Geometry: final body of the model. Coordinates: model frame, mm. A direction names the side the tool comes from. Give positions to 0.01 mm unless a question says otherwise; leave off trailing zeros. Write each loop counter-clockwise with the first axis right and the second up, starting at its lowest first coordinate (ties: lowest second). Pieces come first, ordered by that corner, then holes.
from build123d import *

# Parameters (mm, degrees)
SKETCH1_W           = 75
SKETCH1_H           = 10
BOSS_EXTRUDE1_DEPTH = 100
SKETCH2_R           = 5
CUT_EXTRUDE1_DEPTH  = 10
FILLET1_R           = 10
SKETCH3_R           = 4
CUT_EXTRUDE2_DEPTH  = 192


with BuildPart() as part:
    # Sketch1 → Boss-Extrude1 (new body)
    with BuildSketch(Plane.XY):
        with Locations((112.5, -5)):
            Rectangle(SKETCH1_W, SKETCH1_H)
        with Locations((37.5, -5)):
            Rectangle(SKETCH1_W, SKETCH1_H)
        Polygon((150, 0), (150, -10), (160, -10), (160, 90), (150, 90), align=None)
        Polygon((-10, -10), (0, -10), (0, 0), (0, 90), (-10, 90), align=None)
    extrude(amount=BOSS_EXTRUDE1_DEPTH)

    # Sketch2 → Cut-Extrude1 (cut)
    with BuildSketch(Plane(origin=(0, 0, 0), x_dir=(1, 0, 0), z_dir=(0, 1, 0))):
        with Locations(Location((75, -50, 0), (0, 0, 270))):
            Circle(SKETCH2_R)
    extrude(amount=-CUT_EXTRUDE1_DEPTH, mode=Mode.SUBTRACT)

    # Fillet1
    fillet1_edges = [part.edges().sort_by_distance(p)[0] for p in [
        (160, -10, 50),
        (-10, -10, 50),
    ]]
    fillet(fillet1_edges, radius=FILLET1_R)

    # Sketch3 → Cut-Extrude2 (cut)
    with BuildSketch(Plane.ZY.offset(10)):
        with Locations((50, 65)):
            Circle(SKETCH3_R)
    extrude(amount=-CUT_EXTRUDE2_DEPTH, mode=Mode.SUBTRACT)


solid = part.part
Q1. Section C-C on y = 65. Output: boundary loops of the cut face in (x, z), plus the area to 3 significant figures.
Filled sheet:
outline: (-10, 0) - (0, 0) - (0, 46) - (-10, 46) - close; (-10, 54) - (0, 54) - (0, 100) - (-10, 100) - close; (150, 0) - (160, 0) - (160, 46) - (150, 46) - close; (150, 54) - (160, 54) - (160, 100) - (150, 100) - close
area: 1,840 mm2
Q2. Ray query, line 1 along X through (y, z) = (50, 20.5); line 2 along Y through (x, z) = (152, 50); line 3 along Y through (x, z) = (1.5, 15). Return the intervals inside material, ascending.
Filled sheet:
line 1: x = -10 to 0, 150 to 160
line 2: y = -9.8 to 61, 69 to 90
line 3: y = -10 to 0
Q3. Section A-A on x = 75. Output: boundary loops of the cut face in (y, z).
Filled sheet:
outline: (-10, 0) - (0, 0) - (0, 45) - (-10, 45) - close; (-10, 55) - (0, 55) - (0, 100) - (-10, 100) - close
Q4. Section D-D on y = 39.5. Output: boundary loops of the cut face in (x, z).
Filled sheet:
outline: (-10, 0) - (0, 0) - (0, 100) - (-10, 100) - close; (150, 0) - (160, 0) - (160, 100) - (150, 100) - close
Q5. Section B-B on z = 50. Output: boundary loops of the cut face in (x, y), plus the area to 3 significant figures.
Filled sheet:
outline: (-10, 0) arc R10 ccw to (0, -10) - (70, -10) - (70, 0) - (0, 0) - (0, 61) - (-10, 61) - close; (-10, 69) - (0, 69) - (0, 90) - (-10, 90) - close; (80, -10) - (150, -10) arc R10 ccw to (160, 0) - (160, 61) - (150, 61) - (150, 0) - (80, 0) - close; (150, 69) - (160, 69) - (160, 90) - (150, 90) - close
area: 3,200 mm2
Q6. Access query for faces 4 (the cylindrical face through (70.12, -4.93, 48.92)), 5 (the flat face through (76, 0, 38)). Directions: +Z, -Z, +X, -X, +Y, -Y. A direction counts if a zero-diameter tool reaches every point of the face in a straight line with its end or side. Return the directions, or none.
Filled sheet:
face 4: +Y, -Y
face 5: +Z, -Z, +Y
Q7. Pin query (flat end, axial travel): P1, Ø10, axis at x = 80, z = 60, coming from the +Y side. Return the tip coordinate at first contact, or that it passes through.
Filled sheet:
P1: stops at y = 0
Q8. Pull-direction query (X, two-part tool) for faces 1 (the cylindrical face through (-7.15, -6.99, 50.7)), 2 (the flat face through (150, 46, 49)), 3 (the flat face through (160, 44, 49)); classes: released by +X, released by -X, zero draft, split by the parting line, or undercut.
Filled sheet:
face 1: released by -X
face 2: undercut
face 3: released by +X
